Read the model definition and answer for the solid it produces. Units are mm, in the model's axes. A direction names the side the tool comes from. Round coordinates to 2 decimals unless told otherwise and drop trailing zeros. Loops run counter-clockwise (first coordinate to the right, second up) from the corner with the lowest first, then second, coordinate; pieces in that order, holes last. Notation, with made-up numbers: M 31.5,30.5 L 70.5,30.5 A25 ccw 70.5,66.5 Z; hole C 69.5,52.25 d6. An arc over 180 degrees is marked long. Answer as CSV lines item,"result".
```python
from build123d import *

# Parameters (mm, degrees)
F1_DEPTH = 5
F2_DEPTH = 15


with BuildPart() as f1:
    # F0 (on Top) → F1 (new body)
    with BuildSketch(Plane.XY):
        with BuildLine():
            ThreePointArc((40, 62.5), (37.071068, 69.571068), (30, 72.5))
            Line((30, 72.5), (-30, 72.5))
            ThreePointArc((-30, 72.5), (-37.071068, 69.571068), (-40, 62.5))
            Line((-40, 62.5), (-40, -72.5))
            Line((-40, -72.5), (40, -72.5))
            Line((40, -72.5), (40, 62.5))
        make_face()
        with BuildLine():
            Line((-25, 70), (25, 70))
            ThreePointArc((25, 70), (32.071068, 67.071068), (35, 60))
            Line((35, 60), (35, -55))
            ThreePointArc((35, -55), (33.535534, -58.535534), (30, -60))
            ThreePointArc((30, -60), (26.464466, -61.464466), (25, -65))
            ThreePointArc((25, -65), (23.535534, -68.535534), (20, -70))
            Line((20, -70), (-20, -70))
            ThreePointArc((-20, -70), (-23.535534, -68.535534), (-25, -65))
            ThreePointArc((-25, -65), (-26.464466, -61.464466), (-30, -60))
            ThreePointArc((-30, -60), (-33.535534, -58.535534), (-35, -55))
            Line((-35, -55), (-35, 60))
            ThreePointArc((-35, 60), (-32.071068, 67.071068), (-25, 70))
        make_face(mode=Mode.SUBTRACT)
        with BuildLine():
            ThreePointArc((35, 60), (32.071068, 67.071068), (25, 70))
            Line((25, 70), (-25, 70))
            ThreePointArc((-25, 70), (-32.071068, 67.071068), (-35, 60))
            Line((-35, 60), (-35, -55))
            ThreePointArc((-35, -55), (-33.535534, -58.535534), (-30, -60))
            ThreePointArc((-30, -60), (-26.464466, -61.464466), (-25, -65))
            ThreePointArc((-25, -65), (-23.535534, -68.535534), (-20, -70))
            Line((-20, -70), (20, -70))
            ThreePointArc((20, -70), (23.535534, -68.535534), (25, -65))
            ThreePointArc((25, -65), (26.464466, -61.464466), (30, -60))
            ThreePointArc((30, -60), (33.535534, -58.535534), (35, -55))
            Line((35, -55), (35, 60))
        make_face()
        with BuildLine():
            ThreePointArc((20, -45), (17.071068, -52.071068), (10, -55))
            Line((10, -55), (-10, -55))
            ThreePointArc((-10, -55), (-17.071068, -52.071068), (-20, -45))
            Line((-20, -45), (-20, -15))
            ThreePointArc((-20, -15), (-17.071068, -7.928932), (-10, -5))
            Line((-10, -5), (10, -5))
            ThreePointArc((10, -5), (17.071068, -7.928932), (20, -15))
            Line((20, -15), (20, -45))
        make_face(mode=Mode.SUBTRACT)
        with BuildLine():
            Line((-10, 55), (10, 55))
            ThreePointArc((10, 55), (17.071068, 52.071068), (20, 45))
            Line((20, 45), (20, 15))
            ThreePointArc((20, 15), (17.071068, 7.928932), (10, 5))
            Line((10, 5), (-10, 5))
            ThreePointArc((-10, 5), (-17.071068, 7.928932), (-20, 15))
            Line((-20, 15), (-20, 45))
            ThreePointArc((-20, 45), (-17.071068, 52.071068), (-10, 55))
        make_face(mode=Mode.SUBTRACT)
    extrude(amount=-F1_DEPTH)

    # F0 (on Top) → F2 (join)
    with BuildSketch(Plane.XY):
        with BuildLine():
            ThreePointArc((40, 62.5), (37.071068, 69.571068), (30, 72.5))
            Line((30, 72.5), (-30, 72.5))
            ThreePointArc((-30, 72.5), (-37.071068, 69.571068), (-40, 62.5))
            Line((-40, 62.5), (-40, -72.5))
            Line((-40, -72.5), (40, -72.5))
            Line((40, -72.5), (40, 62.5))
        make_face()
        with BuildLine():
            Line((-25, 70), (25, 70))
            ThreePointArc((25, 70), (32.071068, 67.071068), (35, 60))
            Line((35, 60), (35, -55))
            ThreePointArc((35, -55), (33.535534, -58.535534), (30, -60))
            ThreePointArc((30, -60), (26.464466, -61.464466), (25, -65))
            ThreePointArc((25, -65), (23.535534, -68.535534), (20, -70))
            Line((20, -70), (-20, -70))
            ThreePointArc((-20, -70), (-23.535534, -68.535534), (-25, -65))
            ThreePointArc((-25, -65), (-26.464466, -61.464466), (-30, -60))
            ThreePointArc((-30, -60), (-33.535534, -58.535534), (-35, -55))
            Line((-35, -55), (-35, 60))
            ThreePointArc((-35, 60), (-32.071068, 67.071068), (-25, 70))
        make_face(mode=Mode.SUBTRACT)
    extrude(amount=-F2_DEPTH)


solid = f1.part
```
1) Determine the mould class of faces 4 (the cylindrical face through (17.15, -51.99, -2.46)), 5 (the cylindrical face through (-16.99, 7.85, -2.46)), 6 (the flat face through (-36, 0, -15)), 7 (the cylindrical face through (-36.99, 69.65, -7.4)) for opening direction Y: released by +Y, released by -Y, zero draft, split by the parting line, or undercut.
Evaluation:
face 4,"undercut"
face 5,"undercut"
face 6,"zero draft"
face 7,"released by +Y"
2) Find section B-B, the plane x = 5.5. Give the vertices of the cut face in (y, z).
Evaluation:
outline,"M -72.5,-15 L -70,-15 L -70,-5 L -55,-5 L -55,0 L -72.5,0 Z; M -5,-5 L 5,-5 L 5,0 L -5,0 Z; M 55,-5 L 70,-5 L 70,-15 L 72.5,-15 L 72.5,0 L 55,0 Z"
3) A tool of negligible diameter and unlimited length cuts with its end or side. For faces 1 (the flat face through (35, 3, -10)), 2 (the flat face through (-40, -4, -7)), 3 (the flat face through (20, -30, -2)), from which of +Z, -Z, +X, -X, +Y, -Y can it reach the whole face along a straight path? Write none if from no direction.
Evaluation:
face 1,"-Z"
face 2,"+Z, -Z, -X, +Y, -Y"
face 3,"+Z, -Z"
4) Find section A-A, the plane y = 39.5. Give the vertices of the cut face in (x, z), then the cut area to 3 significant figures.
Evaluation:
outline,"M -40,-15 L -35,-15 L -35,-5 L -20,-5 L -20,0 L -40,0 Z; M 20,-5 L 35,-5 L 35,-15 L 40,-15 L 40,0 L 20,0 Z"
area,"300 mm^2"
5) Find section D-D, the plane x = -18. Give the vertices of the cut face in (y, z).
Evaluation:
outline,"M -72.5,-15 L -70,-15 L -70,-5 L -51,-5 L -51,0 L -72.5,0 Z; M -9,-5 L 9,-5 L 9,0 L -9,0 Z; M 51,-5 L 70,-5 L 70,-15 L 72.5,-15 L 72.5,0 L 51,0 Z"
6) Straight lines are drawn through the part: line 1 (Y direction, x = -3, z = -3.25); line 2 (X direction, y = 2, z = -12); line 3 (X direction, y = 25, z = -1.5). For each, find the intervals that lie inside material, in ascending order.
Evaluation:
line 1,"y = -72.5 to -55, -5 to 5, 55 to 72.5"
line 2,"x = -40 to -35, 35 to 40"
line 3,"x = -40 to -20, 20 to 40"
7) This flat-tipped pin is pushed along its axis until it touches: P1, Ø12, axis at x = -15, y = 44, coming from the -Z side. Where does it stop, or does it pass through?
Evaluation:
P1,"stops at z = -5"
8) Find section C-C, the plane z = -11. Give the vertices of the cut face in (x, y), then the cut area to 3 significant figures.
Evaluation:
outline,"M -40,-72.5 L 40,-72.5 L 40,62.5 A10 ccw 30,72.5 L -30,72.5 A10 ccw -40,62.5 Z; hole M -35,-55 A5 ccw -30,-60 A5 cw -25,-65 A5 ccw -20,-70 L 20,-70 A5 ccw 25,-65 A5 cw 30,-60 A5 ccw 35,-55 L 35,60 A10 ccw 25,70 L -25,70 A10 ccw -35,60 Z"
area,"2,010 mm^2"
